```python
from build123d import *

# Parameters (mm, degrees)
BOSS_EXTRUDE1_DEPTH      = 15
SKETCH2_R                = 2
CUT_EXTRUDE1_DEPTH       = 1
CUT_EXTRUDE1_DEPTH_BACK  = 16
SKETCH3_W                = 30
SKETCH3_H                = 7
BOSS_EXTRUDE2_DEPTH      = 5
BOSS_EXTRUDE2_DEPTH_BACK = 15
SKETCH4_W                = 38.205528846
SKETCH4_H                = 30.397050351
CUT_EXTRUDE2_DEPTH       = 6
CUT_EXTRUDE2_DEPTH_BACK  = 16
SKETCH5_R                = 2.5
BOSS_EXTRUDE3_DEPTH      = 15


with BuildPart() as part:
    # Sketch1 → Boss-Extrude1 (new body)
    with BuildSketch(Plane.XY):
        with BuildLine():
            Line((-12.914434136, 15.27145674), (32.740581269, 53.879999426))
            ThreePointArc((32.740581269, 53.879999426), (53.033008589, 53.033008589), (53.879999426, 32.740581269))
            Line((53.879999426, 32.740581269), (15.27145674, -12.914434136))
            ThreePointArc((15.27145674, -12.914434136), (-14.142135624, -14.142135624), (-12.914434136, 15.27145674))
        make_face()
    extrude(amount=BOSS_EXTRUDE1_DEPTH)

    # Sketch2 → Cut-Extrude1 (cut, two sides)
    with BuildSketch(Plane.XY.offset(15)) as cut_extrude1_sk:
        Circle(SKETCH2_R)
        with Locations((42.426406871, 42.426406871)):
            Circle(SKETCH2_R)
    extrude(amount=CUT_EXTRUDE1_DEPTH, mode=Mode.SUBTRACT)
    extrude(cut_extrude1_sk.sketch, amount=-CUT_EXTRUDE1_DEPTH_BACK, mode=Mode.SUBTRACT)

    # Sketch3 → Boss-Extrude2 (add, two sides)
    with BuildSketch(Plane.XY.offset(15)) as boss_extrude2_sk:
        with Locations((0, 13)):
            Rectangle(SKETCH3_W, SKETCH3_H)
    extrude(amount=BOSS_EXTRUDE2_DEPTH)
    extrude(boss_extrude2_sk.sketch, amount=-BOSS_EXTRUDE2_DEPTH_BACK)

    # Sketch4 → Cut-Extrude2 (cut, two sides)
    with BuildSketch(Plane.XY.offset(15)) as cut_extrude2_sk:
        with Locations((-4.102764423, 31.698525176)):
            Rectangle(SKETCH4_W, SKETCH4_H)
    extrude(amount=CUT_EXTRUDE2_DEPTH, mode=Mode.SUBTRACT)
    extrude(cut_extrude2_sk.sketch, amount=-CUT_EXTRUDE2_DEPTH_BACK, mode=Mode.SUBTRACT)

    # Sketch5 → Boss-Extrude3 (add)
    with BuildSketch(Plane(origin=(0, 16.5, 0), x_dir=(1, 0, 0), z_dir=(0, 1, 0))):
        with Locations((0, -10)):
            Circle(SKETCH5_R)
    extrude(amount=BOSS_EXTRUDE3_DEPTH)


solid = part.part
```
CAD build for the part. Positions are in the model's coordinates, mm. A direction names the side the tool comes from. Give positions to 0.01 mm unless a question says otherwise; leave off trailing zeros. Write each loop counter-clockwise with the first axis right and the second up, starting at its lowest first coordinate (ties: lowest second). Pieces come first, ordered by that corner, then holes. Notation, with made-up numbers: M 64,7.25 L 105,7.25 A33 ccw 105,41.25 Z; hole C 10.25,59.5 d11. An arc over 180 degrees is marked long. Return JSON: item names as keys, results as strings. Group by question number.
(1) Band-saw the part on C-C (y = 18.5). Give the cut face in (x, z).
(2) Flat gauge pins, fed straight in: pin 1 Ø5 at (x, z) = (-8.5, 5.5) entering from -Y; pin 2 Ø2.5 at (x, z) = (2, 18) entering from -Y; pin 3 Ø5.5 at (x, z) = (-1, 9.5) entering from +Y; pin 4 Ø2.5 at (x, y) = (42.43, 42.43) entering from +Z. Where does each tip first touch, or does it go through?
(3) Band-saw the part on A-A (x = 0). Give the cut face in (y, z).
(4) Mould opens along X. For faces 4 (the face through (34.846, 10.233, 7.395)), 5 (the face through (0, 13, 20)), 6 (the face through (44.274, 41.66, 7.605)), 7 (the face through (0, -2, 8)) say: pulls with the +X half, pulls with the -X half, needs draft (parallel to the pull), parting line crosses it, or undercut.
(5) Band-saw the part on D-D (z = 2.5). Give the cut face in (x, y), and give its area (3 significant figures).
(6) Drill centre lines: L1, parallel to Y at x = 0, z = 9.75; L2, parallel to Y at x = 0, z = 5; L3, parallel to Z at x = 50.5, y = 37.5. Where is each one in solid material? Low to high. Write a range as [from, to].
(7) 3-axis set-ups, long thin cutter, end or side, ignore diameter. For faces 1 (the face through (-15, 15, 12)), 2 (the face through (0, 9.5, 17)), 3 (the face through (0, 31.5, 10)): which of +Z, -Z, +X, -X, +Y, -Y reach the whole face in a straight line?
(8) Band-saw the part on B-B (z = 10). Give the cut face in (x, y), and give its area (3 significant figures).
Entries:
{
 "1": {"outline": "C 0,10 d5; M 15,0 L 41.84,0 L 41.84,15 L 15,15 Z"},
 "2": {"pin 1": "stops at y = -19.08", "pin 2": "stops at y = 9.5", "pin 3": "stops at y = 31.5", "pin 4": "passes through"},
 "3": {"outline": "M -20,0 L -2,0 L -2,15 L -20,15 Z; M 2,0 L 16.5,0 L 16.5,7.5 L 31.5,7.5 L 31.5,12.5 L 16.5,12.5 L 16.5,20 L 9.5,20 L 9.5,15 L 2,15 Z"},
 "4": {"face 4": "pulls with the +X half", "face 5": "needs draft", "face 6": "undercut", "face 7": "undercut"},
 "5": {"outline": "M -15,13.23 A20 ccw long 15.27,-12.91 L 53.88,32.74 A15 ccw 32.74,53.88 L 15,38.88 L 15,16.5 L -15,16.5 Z; hole C 0,0 d4; hole C 42.43,42.43 d4", "area": "2,770 mm^2"},
 "6": {"L1": "y = [-20, -2], [2, 31.5]", "L2": "y = [-20, -2], [2, 16.5]", "L3": "z = [0, 15]"},
 "7": {"face 1": "+Z, -X, +Y", "face 2": "+Z, +X, -X, -Y", "face 3": "+Z, -Z, -X, +Y"},
 "8": {"outline": "M -15,13.23 A20 ccw long 15.27,-12.91 L 53.88,32.74 A15 ccw 32.74,53.88 L 15,38.88 L 15,16.5 L 2.5,16.5 L 2.5,31.5 L -2.5,31.5 L -2.5,16.5 L -15,16.5 Z; hole C 0,0 d4; hole C 42.43,42.43 d4", "area": "2,850 mm^2"}
}
